from build123d import *

# Parameters (mm, degrees)
F1_DEPTH    = 2.75
F2_DEPTH    = 0.6
F3_SIZE     = 2
F4_W        = 6.5
F4_H        = 27.2
F5_DEPTH    = 1.2
F6_C1_SIZE2 = 4
F6_C1_SIZE  = 1.1
F6_C2_SIZE2 = 1.1
F6_C2_SIZE  = 4
F7_C1_SIZE2 = 1.1
F7_C1_SIZE  = 10
F7_C2_SIZE2 = 10
F7_C2_SIZE  = 1.1


# Not quite as in the source:
# - a pattern or mirror of a feature is missing from the dataset's text; its kind, count and spacing are read off the source's solid


with BuildPart() as f1:
    # F0 (on Top) → F1 (new body, symmetric)
    with BuildSketch(Plane.XY):
        Polygon((3.25, 30), (0, 30), (-3.25, 30), (-3.25, 21), (-3.25, 7.8), (-3.25, 2.8), (-8.25, 2.8), (-11, 2.8), (-11.1000184963, 8), (-11.25, 15.7975959316), (-13.2, 19.5), (-13.2, 22.5), (-15, 22.5), (-15.75, 15.5), (-14.75, 12.5), (-13.75, 13.5), (-14, 0), (0, 0), (14, 0), (13.75, 13.5), (14.75, 12.5), (15.75, 15.5), (15, 22.5), (13.2, 22.5), (13.2, 19.5), (11.25, 15.7975959316), (11.1000184963, 8), (11, 2.8), (8.25, 2.8), (3.25, 2.8), (3.25, 7.8), (3.25, 21), align=None)
    extrude(amount=F1_DEPTH, both=True)

    # F0 (on Top) → F2 (join, symmetric)
    with BuildSketch(Plane.XY):
        with BuildLine():
            Line((-11.25, 15.7975959316), (-11.1000184963, 8))
            Line((-11.1000184963, 8), (-7.75, 14))
            Line((-7.75, 14), (-7.75, 18))
            Line((-7.75, 18), (-8.25, 18))
            ThreePointArc((-8.25, 18), (-8.9571067812, 18.2928932188), (-9.25, 19))
            Line((-9.25, 19), (-9.25, 28))
            Line((-9.25, 28), (-12.75, 28))
            Line((-12.75, 28), (-15, 22.5))
            Line((-15, 22.5), (-13.2, 22.5))
            Line((-13.2, 22.5), (-13.2, 19.5))
            Line((-13.2, 19.5), (-11.25, 15.7975959316))
        make_face()
        Polygon((-3.25, 21), (-3.25, 30), (-5.25, 21), align=None)
        Polygon((5.25, 21), (3.25, 30), (3.25, 21), align=None)
        with BuildLine():
            Line((7.75, 14), (11.1000184963, 8))
            Line((11.1000184963, 8), (11.25, 15.7975959316))
            Line((11.25, 15.7975959316), (13.2, 19.5))
            Line((13.2, 19.5), (13.2, 22.5))
            Line((13.2, 22.5), (15, 22.5))
            Line((15, 22.5), (12.75, 28))
            Line((12.75, 28), (9.25, 28))
            Line((9.25, 28), (9.25, 19))
            ThreePointArc((9.25, 19), (8.9571067812, 18.2928932188), (8.25, 18))
            Line((8.25, 18), (7.75, 18))
            Line((7.75, 18), (7.75, 14))
        make_face()
        with BuildLine():
            ThreePointArc((8.25, 2.8), (4.7144660941, 4.2644660941), (3.25, 7.8))
            Line((3.25, 7.8), (3.25, 2.8))
            Line((3.25, 2.8), (8.25, 2.8))
        make_face()
        with BuildLine():
            Line((-3.25, 2.8), (-3.25, 7.8))
            ThreePointArc((-3.25, 7.8), (-4.7144660941, 4.2644660941), (-8.25, 2.8))
            Line((-8.25, 2.8), (-3.25, 2.8))
        make_face()
    extrude(amount=F2_DEPTH, both=True)

    # F3
    f3_edges = [f1.edges().sort_by_distance(p)[0] for p in [
        (14.1, 22.5, 2.75),
        (14.1, 22.5, -2.75),
        (-14.1, 22.5, 2.75),
        (-14.1, 22.5, -2.75),
    ]]
    chamfer(f3_edges, length=F3_SIZE)

    # F4 (on face) → F5 (join)
    with BuildSketch(Plane.XY.offset(2.75)):
        with Locations((0, 16.4)):
            Rectangle(F4_W, F4_H)
    f5 = extrude(amount=F5_DEPTH)

    # F5_copies: F5 across plane
    add(f5.mirror(Plane(origin=(0, 0, 0), x_dir=(-1, 0, 0), z_dir=(0, 0, -1))))

    # F6: chamfer of 4 x 1.1 on 2 edges, made by hand

    # F6_c1
    f6_c1_edges = [f1.edges().sort_by_distance(p)[0] for p in [
        (0, 2.8, -3.95),
    ]]
    f6_c1_side = f1.faces().sort_by_distance((0, 2.8, -3.928))[0]
    chamfer(f6_c1_edges, length=F6_C1_SIZE, length2=F6_C1_SIZE2, reference=f6_c1_side)

    # F6_c2
    f6_c2_edges = [f1.edges().sort_by_distance(p)[0] for p in [
        (0, 2.8, 3.95),
    ]]
    f6_c2_side = f1.faces().sort_by_distance((0, 2.822, 3.95))[0]
    chamfer(f6_c2_edges, length=F6_C2_SIZE, length2=F6_C2_SIZE2, reference=f6_c2_side)

    # F7: chamfer of 1.1 x 10 on 2 edges, made by hand

    # F7_c1
    f7_c1_edges = [f1.edges().sort_by_distance(p)[0] for p in [
        (0, 30, 3.95),
    ]]
    f7_c1_side = f1.faces().sort_by_distance((0, 29.978, 3.95))[0]
    chamfer(f7_c1_edges, length=F7_C1_SIZE, length2=F7_C1_SIZE2, reference=f7_c1_side)

    # F7_c2
    f7_c2_edges = [f1.edges().sort_by_distance(p)[0] for p in [
        (0, 30, -3.95),
    ]]
    f7_c2_side = f1.faces().sort_by_distance((0, 30, -3.928))[0]
    chamfer(f7_c2_edges, length=F7_C2_SIZE, length2=F7_C2_SIZE2, reference=f7_c2_side)


solid = f1.part
Geometry: final body of the model. Coordinates: model frame, mm. A direction names the side the tool comes from. Round coordinates to 2 decimals unless told otherwise and drop trailing zeros. Order: outer loops, then holes, each group sorted by start corner. A loop starts at its lowest first (then second) coordinate and runs counter-clockwise, first axis right, second up. Notation, with made-up numbers: (-14, -3.75) -> (12, -3.75) arc R16 ccw to (12, 5.25) -> close; hole circle Ø2 at (-37, 21.5). An arc over 180 degrees is marked (long way). Put each result on its own line as item: value. Start each with the question number.
Q1. First-contact query: pin 1 (1.5 mm diameter, centred on x = -5.5, y = 21, fed in from -Z); pin 2 (1 mm diameter, centred on x = 10.5, z = 0, fed in from +Y); pin 3 (2 mm diameter, centred on y = 7, z = 0, fed in from +X). Flat tips, straight axial feed; report the tip coordinate or a pass-through.
Q2. Section C-C on x = 0.5. Return the cut outline in (y, z).
Q3. Pull-direction query (Y, two-part tool) for faces 6 (the flat face through (0, 4.8, 3.4)), 7 (the cylindrical face through (-5, 4, 0)), 8 (the flat face through (9.25, 24, 0)); classes: +Y half, -Y half, draft (parallel to the pull), parting line (faces both ways), or undercut.
Q4. Section B-B on x = -10. Return the cut outline in (y, z), and give its area (3 significant figures).
Q5. Section D-D on z = 1.25. Return the cut outline in (x, y).
Q6. Line query: probe 1 along X at (y, z) = (17, 0.5); probe 2 along X at (y, z) = (12, 1.25); probe 3 along Z at (x, y) = (-8, 1.75). Output: solid intervals per line, ascending.
Q7. Section A-A on y = 25.75. Return the cut outline in (x, z), and give its area (3 significant figures).
Q8. Reachability of faces 1 (the flat face through (14.22, 21.51, 1.74)), 2 (the flat face through (4.264, 25.437, -0.008)), 3 (the flat face through (-4, 24, 0.6)), 4 (the flat face through (-9.448, 10.958, -0.008)), 5 (the flat face through (-4, 24, -0.6)) from +Z, -Z, +X, -X, +Y, -Y: full face, straight path, thin tool, end or side. Return the list, or none.
Ans:
1. pin 1: stops at z = -0.6
1. pin 2: stops at y = 28
1. pin 3: stops at x = 13.89
2. outline: (0, -2.75) -> (2.8, -2.75) -> (2.8, -2.85) -> (6.8, -3.95) -> (20, -3.95) -> (30, -2.85) -> (30, 2.85) -> (20, 3.95) -> (6.8, 3.95) -> (2.8, 2.85) -> (2.8, 2.75) -> (0, 2.75) -> close
3. face 6: -Y half
3. face 7: undercut
3. face 8: draft
4. outline: (0, -2.75) -> (2.8, -2.75) -> (2.8, 2.75) -> (0, 2.75) -> close; (9.97, -0.6) -> (28, -0.6) -> (28, 0.6) -> (9.97, 0.6) -> close
4. area: 37.0 mm2
5. outline: (-15.75, 15.5) -> (-14.75, 12.5) -> (-13.75, 13.5) -> (-14, 0) -> (14, 0) -> (13.75, 13.5) -> (14.75, 12.5) -> (15.75, 15.5) -> (15.05, 22) -> (13.2, 22) -> (13.2, 19.5) -> (11.25, 15.8) -> (11, 2.8) -> (3.25, 2.8) -> (3.25, 30) -> (-3.25, 30) -> (-3.25, 2.8) -> (-11, 2.8) -> (-11.25, 15.8) -> (-13.2, 19.5) -> (-13.2, 22) -> (-15.05, 22) -> close
6. probe 1: x = -15.59 to -7.75, -3.25 to 3.25, 7.75 to 15.59
6. probe 2: x = -13.78 to -11.18, -3.25 to 3.25, 11.18 to 13.78
6. probe 3: z = -2.75 to 2.75
7. outline: (-13.67, -0.6) -> (-9.25, -0.6) -> (-9.25, 0.6) -> (-13.67, 0.6) -> close; (-4.19, -0.6) -> (-3.25, -0.6) -> (-3.25, -3.32) -> (3.25, -3.32) -> (3.25, -0.6) -> (4.19, -0.6) -> (4.19, 0.6) -> (3.25, 0.6) -> (3.25, 3.32) -> (-3.25, 3.32) -> (-3.25, 0.6) -> (-4.19, 0.6) -> close; (9.25, -0.6) -> (13.67, -0.6) -> (13.67, 0.6) -> (9.25, 0.6) -> close
7. area: 56.0 mm2
8. face 1: +Z, +X, +Y
8. face 2: +Z, -Z, +Y
8. face 3: +Z, +Y
8. face 4: +Z, -Z
8. face 5: -Z, +Y
